Could you check a few things on this model? Use its own coordinates, in mm. A direction names the side the tool comes from. Coordinates: 2 decimals unless noted, no trailing zeros. Order: outer loops, then holes, each group sorted by start corner. A loop starts at its lowest first (then second) coordinate and runs counter-clockwise, first axis right, second up. Notation, with made-up numbers: (-10.5, 45.25) -> (33.5, 45.25) arc R32 ccw to (33.5, 77.25) -> close; hole circle Ø6 at (-4.5, 86). An arc over 180 degrees is marked (long way). Put each result on its own line as item: value. Start each with the question number.
Q1. Please list where these lines run through material, in increasing order: line 1 along X through (y, z) = (2.5, 0); line 2 along Z through (x, y) = (12.5, 9); line 3 along Y through (x, z) = (-1.5, -11).
Q2. For faces 1 (the face through (-5.643, 4.93, 11.69)), 2 (the face through (-8, 8, 0)), 3 (the face through (-21.414, 3.037, 0.208)), 4 (the face through (19, 4, 0)), 5 (the face through (-3.244, 1.972, -7.721)), which set-ups out of +Z, -Z, +X, -X, +Y, -Y let a thin tool reach every point of the face, with its end or its side?
Q3. If we section it at B-B (y = 1.25): Please give me the cut outline in (x, z), and give its area (3 significant figures).
Q4. If we section it at C-C (x = -18.5): Please give me the cut outline in (y, z), and give its area (4 significant figures).
Q5. If we section it at A-A (x = 0): Please give me the cut outline in (y, z).
Q6. We'd pull the mould along Z, two halves only. Please class faces 6 (the face through (16, 5, -7)), 7 (the face through (17, 5, 7)), 8 (the face through (8.89, 6.14, 3.45)): +Z half, -Z half, draft (parallel to the pull), parting line (faces both ways), or undercut.
Q7. Will these pins go through, and if not, where does the flat tip stop? pin 1 (1.9 mm diameter, centred on x = -23, z = 0, fed in from -Y); pin 2 (4 mm diameter, centred on x = -22, y = 8.5, fed in from +Z); pin 3 (2.5 mm diameter, centred on x = -15, z = 0, fed in from +Y); pin 4 (5.5 mm diameter, centred on x = 19.5, z = 0, fed in from +Y).
from build123d import *

# Parameters (mm, degrees)
ESQUISSE1_R                  = 2
BOSS_EXTRU_1_DEPTH           = 10
ESQUISSE2_W                  = 10.2
ESQUISSE2_H                  = 6
ENL_V_MAT_EXTRU_1_DEPTH      = 20
CHANFREIN1_SIZE              = 2.5
CHANFREIN2_SIZE              = 1.8
CHANFREIN1_OF_SYM_TRIE1_SIZE = 2.5
CHANFREIN2_OF_SYM_TRIE1_SIZE = 1.8
ESQUISSE5_R                  = 1.6
ENL_V_MAT_EXTRU_4_DEPTH      = 7
CHANFREIN4_SIZE              = 2.1
CHANFREIN5_SIZE              = 2
ENL_V_MAT_EXTRU_5_DEPTH      = 4
CHANFREIN6_SIZE              = 4


with BuildPart() as part:
    # Esquisse1 → Boss.-Extru.1 (new body)
    with BuildSketch(Plane(origin=(0, 0, 0), x_dir=(1, 0, 0), z_dir=(0, 1, 0))):
        with BuildLine():
            Line((7, 7), (28, 7))
            Line((28, 7), (28, -7))
            Line((28, -7), (7, -7))
            Line((7, -7), (4.322606063, -16.251030305))
            ThreePointArc((4.322606063, -16.251030305), (0, -19.5), (-4.322606063, -16.251030305))
            Line((-4.322606063, -16.251030305), (-7, -7))
            Line((-7, -7), (-28, -7))
            Line((-28, -7), (-28, 7))
            Line((-28, 7), (-7, 7))
            Line((-7, 7), (-4.322606063, 16.251030305))
            ThreePointArc((-4.322606063, 16.251030305), (0, 19.5), (4.322606063, 16.251030305))
            Line((4.322606063, 16.251030305), (7, 7))
        make_face()
        with Locations(Location((0, 0, 0), (0, 0, 270))):
            Circle(ESQUISSE1_R, mode=Mode.SUBTRACT)
    extrude(amount=BOSS_EXTRU_1_DEPTH)

    # Esquisse2 → Enlèv. mat.-Extru.1 (cut)
    with BuildSketch(Plane.ZY.offset(28)):
        with Locations((0, 7)):
            Rectangle(ESQUISSE2_W, ESQUISSE2_H)
    enl_v_mat_extru_1 = extrude(amount=-ENL_V_MAT_EXTRU_1_DEPTH, mode=Mode.SUBTRACT)

    # Chanfrein1
    chanfrein1_edges = [part.edges().sort_by_distance(p)[0] for p in [
        (-18, 4, -5.1),
        (-18, 4, 5.1),
    ]]
    chamfer(chanfrein1_edges, length=CHANFREIN1_SIZE)

    # Chanfrein2
    chanfrein2_edges = [part.edges().sort_by_distance(p)[0] for p in [
        (-8, 4, 0),
        (-8, 5.25, -3.85),
        (-8, 5.25, 3.85),
    ]]
    chamfer(chanfrein2_edges, length=CHANFREIN2_SIZE)

    # Symétrie1: Enlèv. mat.-Extru.1 across plane
    add(enl_v_mat_extru_1.mirror(Plane(origin=(0, 0, 0), x_dir=(0, 0, 1), z_dir=(1, 0, 0))), mode=Mode.SUBTRACT)

    # Chanfrein1 of Symétrie1
    chanfrein1_of_sym_trie1_edges = [part.edges().sort_by_distance(p)[0] for p in [
        (18, 4, -5.1),
        (18, 4, 5.1),
    ]]
    chamfer(chanfrein1_of_sym_trie1_edges, length=CHANFREIN1_OF_SYM_TRIE1_SIZE)

    # Chanfrein2 of Symétrie1
    chanfrein2_of_sym_trie1_edges = [part.edges().sort_by_distance(p)[0] for p in [
        (8, 4, 0),
        (8, 5.25, -3.85),
        (8, 5.25, 3.85),
    ]]
    chamfer(chanfrein2_of_sym_trie1_edges, length=CHANFREIN2_OF_SYM_TRIE1_SIZE)

    # Esquisse5 → Enlèv. mat.-Extru.4 (cut)
    with BuildSketch(Plane.XZ):
        with Locations(Location((-23, 0, 0), (0, 0, 270))):
            Circle(ESQUISSE5_R)
        with Locations(Location((-13, 0, 0), (0, 0, 270))):
            Circle(ESQUISSE5_R)
        with Locations(Location((13, 0, 0), (0, 0, 270))):
            Circle(ESQUISSE5_R)
        with Locations(Location((23, 0, 0), (0, 0, 270))):
            Circle(ESQUISSE5_R)
    extrude(amount=-ENL_V_MAT_EXTRU_4_DEPTH, mode=Mode.SUBTRACT)

    # Chanfrein4
    chanfrein4_edges = [part.edges().sort_by_distance(p)[0] for p in [
        (-23, 0, 1.6),
        (-13, 0, 1.6),
        (13, 0, 1.6),
        (23, 0, 1.6),
    ]]
    chamfer(chanfrein4_edges, length=CHANFREIN4_SIZE)

    # Chanfrein5
    chanfrein5_edges = [part.edges().sort_by_distance(p)[0] for p in [
        (28, 5, -7),
        (28, 5, 7),
        (-28, 5, -7),
        (-28, 5, 7),
    ]]
    chamfer(chanfrein5_edges, length=CHANFREIN5_SIZE)

    # Esquisse6 → Enlèv. mat.-Extru.5 (cut)
    with BuildSketch(Plane.XZ):
        with BuildLine():
            Line((-3.979949748, -0.4), (-2.487468593, -15.25))
            ThreePointArc((-2.487468593, -15.25), (0, -17.5), (2.487468593, -15.25))
            Line((2.487468593, -15.25), (3.979949748, -0.4))
            ThreePointArc((3.979949748, -0.4), (4, 0), (3.979949748, 0.4))
            Line((3.979949748, 0.4), (2.487468593, 15.25))
            ThreePointArc((2.487468593, 15.25), (0, 17.5), (-2.487468593, 15.25))
            Line((-2.487468593, 15.25), (-3.979949748, 0.4))
            ThreePointArc((-3.979949748, 0.4), (-4, 0), (-3.979949748, -0.4))
        make_face()
    extrude(amount=-ENL_V_MAT_EXTRU_5_DEPTH, mode=Mode.SUBTRACT)

    # Chanfrein6
    chanfrein6_edges = [part.edges().sort_by_distance(p)[0] for p in [
        (0, 10, -2),
    ]]
    chamfer(chanfrein6_edges, length=CHANFREIN6_SIZE)


solid = part.part
The answers:
1. line 1: -28 to -24.6, -21.4 to -14.6, -11.4 to -4, 4 to 11.4, 14.6 to 21.4, 24.6 to 28
1. line 2: -7 to -5.1, 5.1 to 7
1. line 3: 4 to 10
2. face 1: +Z, -X, +Y, -Y
2. face 2: -X, +Y
2. face 3: +Y, -Y
2. face 4: +X, +Y
2. face 5: -Y
3. outline: (-28, -5) -> (-26, -7) -> (-7, -7) -> (-4.32, -16.25) arc R4.5 ccw to (4.32, -16.25) -> (7, -7) -> (26, -7) -> (28, -5) -> (28, 5) -> (26, 7) -> (7, 7) -> (4.32, 16.25) arc R4.5 ccw to (-4.32, 16.25) -> (-7, 7) -> (-26, 7) -> (-28, 5) -> close; hole circle Ø4.9 at (-23, 0); hole circle Ø4.9 at (-13, 0); hole (-3.98, -0.4) -> (-2.49, -15.25) arc R2.5 ccw to (2.49, -15.25) -> (3.98, -0.4) arc R4 ccw to (3.98, 0.4) -> (2.49, 15.25) arc R2.5 ccw to (-2.49, 15.25) -> (-3.98, 0.4) arc R4 ccw to start; hole circle Ø4.9 at (13, 0); hole circle Ø4.9 at (23, 0)
3. area: 736 mm^2
4. outline: (0, -7) -> (10, -7) -> (10, -5.1) -> (6.5, -5.1) -> (4, -2.6) -> (4, 2.6) -> (6.5, 5.1) -> (10, 5.1) -> (10, 7) -> (0, 7) -> close
4. area: 85.05 mm^2
5. outline: (0, -19.5) -> (10, -19.5) -> (10, -6) -> (6, -2) -> (4, -2) -> (4, -17.5) -> (0, -17.5) -> close; (0, 17.5) -> (4, 17.5) -> (4, 2) -> (6, 2) -> (10, 6) -> (10, 19.5) -> (0, 19.5) -> close
6. face 6: -Z half
6. face 7: +Z half
6. face 8: undercut
7. pin 1: through
7. pin 2: z = 7
7. pin 3: y = 4
7. pin 4: y = 4.15
